Drawing for the job (mm, zero at the part's lowest x, y, z). A direction names the side the tool comes from. Coordinates: 2 decimals unless noted, no trailing zeros. Loops run counter-clockwise (first coordinate to the right, second up) from the corner with the lowest first, then second, coordinate; pieces in that order, holes last. Notation, with made-up numbers: (-7, 24) - (27, 24) arc R24 ccw to (27, 50) - close; hole circle Ø5 at (72.25, 27). An arc over 180 degrees is marked (long way). One line per item, written item: value.
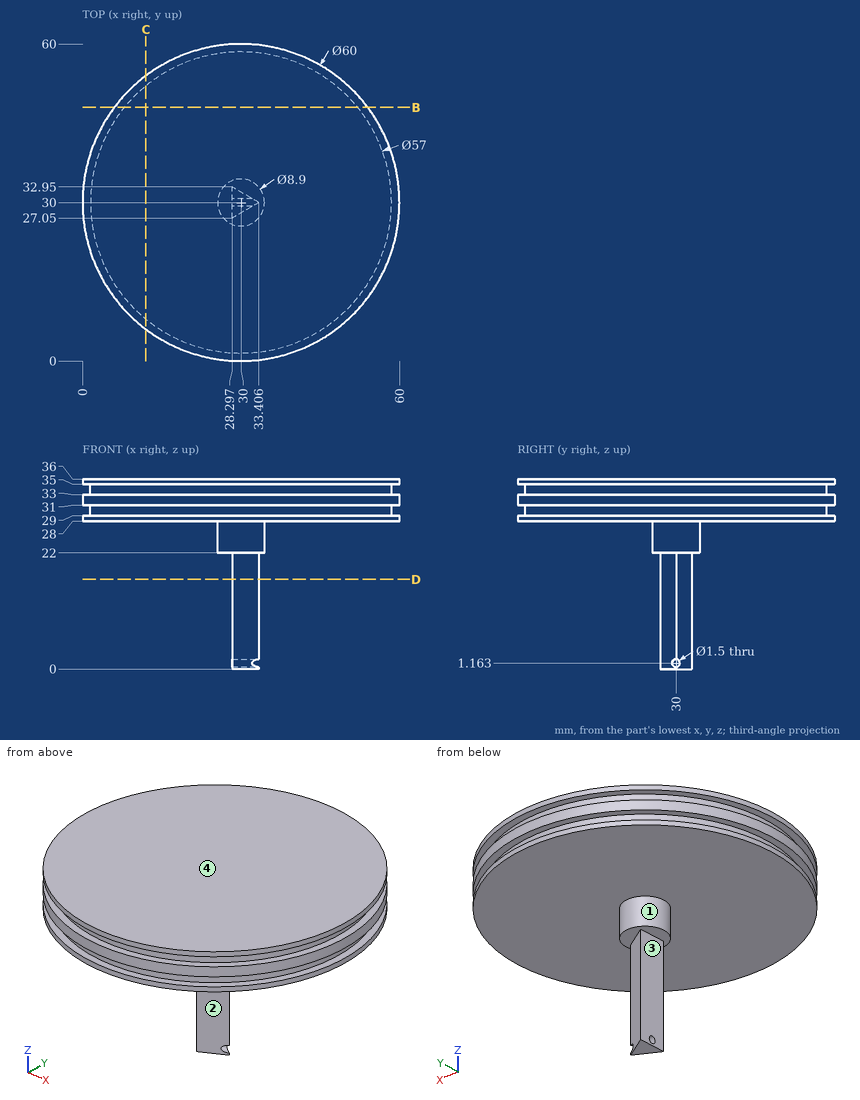
Item 1: Tool access for the marked faces 1, 2, 3 and 4: list every direction of +Z, -Z, +X, -X, +Y, -Y with a clear straight run to the whole face (end or side of a thin tool).
Check result:
face 1: -Z
face 2: -Z, +X, -Y
face 3: -Z, -X, +Y, -Y
face 4: +Z, +X, -X, +Y, -Y
Item 2: Probe probe 1 along Z at (x, y) = (57, 42); probe 2 along Z at (x, y) = (31.2, 30); probe 3 along Z at (x, y) = (36.5, 56). List the from-to ranges inside material, lowest first. Write a range as from..to.
Check result:
probe 1: z = 28..29, 31..33, 35..36
probe 2: z = 0..0.41, 1.91..36
probe 3: z = 28..36
Item 3: Cut at B-B, the plane y = 48. Write the cut outline in (x, z).
Check result:
outline: (6, 28) - (54, 28) - (54, 29) - (52.1, 29) - (52.1, 31) - (54, 31) - (54, 33) - (52.1, 33) - (52.1, 35) - (54, 35) - (54, 36) - (6, 36) - (6, 35) - (7.9, 35) - (7.9, 33) - (6, 33) - (6, 31) - (7.9, 31) - (7.9, 29) - (6, 29) - close
Item 4: Drop flat-ended pins along their axis: P1, Ø12, axis at x = 34, z = 32, coming from the -Y side; P2, Ø10, axis at x = 39.5, z = 5.5, coming from the -Y side; P3, Ø1.5, axis at y = 28.5, z = 4.5, coming from the +X side (1 decimal); P4, Ø6, axis at x = 24, y = 25, coming from the -Z side. Give the stop position or say it passes through.
Check result:
P1: stops at y = 0
P2: passes through
P3: stops at x = 32.1
P4: stops at z = 28
Item 5: Cut at D-D, the plane z = 17. Write the cut outline in (x, y).
Check result:
outline: (28.3, 27.05) - (33.41, 30) - (28.3, 32.95) - close
